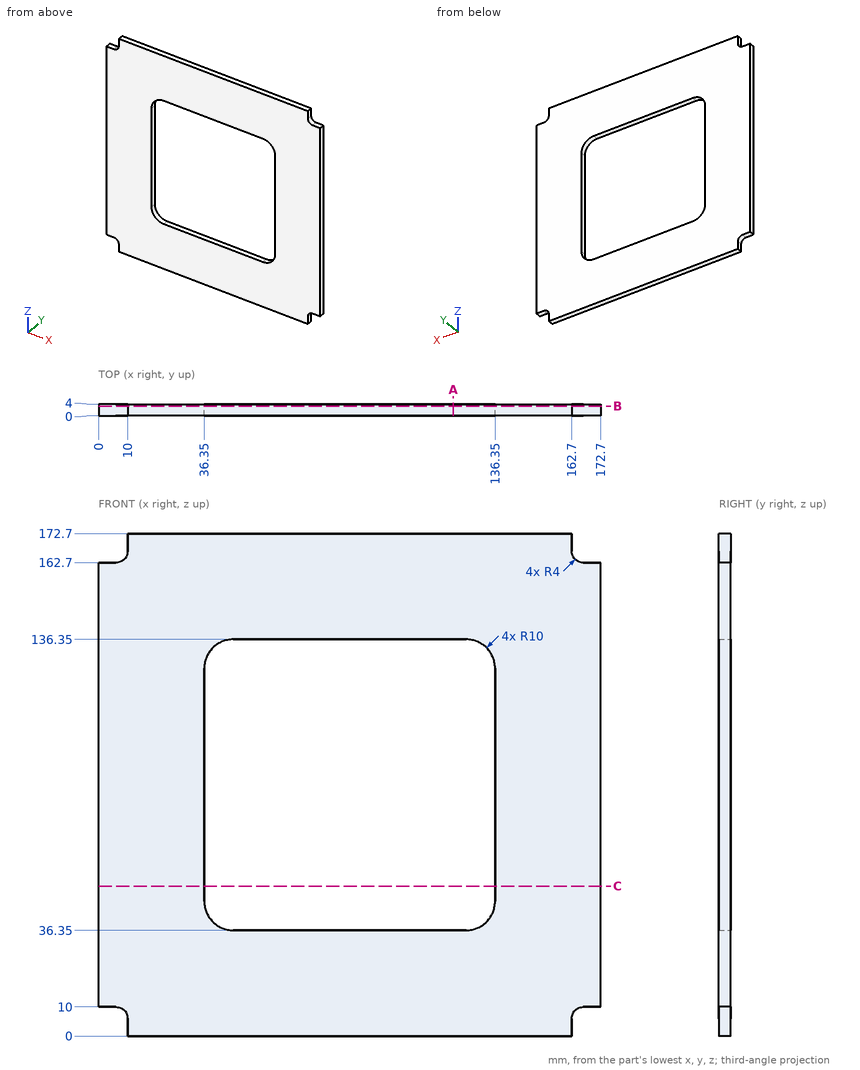
Verification items for this drawing (mm, ordinates from the low corner). Coordinates: 2 decimals unless noted, no trailing zeros. Order: outer loops, then holes, each group sorted by start corner. A loop starts at its lowest first (then second) coordinate and runs counter-clockwise, first axis right, second up. Notation, with made-up numbers: M 44.5,40 L 78.5,40 A25 cw 78.5,78 Z; hole C -4.75,66 d8. An arc over 180 degrees is marked long. One line per item, written item: value. Start each with the question number.
Item 1: Thickness scan on probe 1 along X at (y, z) = (3.35, 97); probe 2 along Z at (x, y) = (42, 2.2). Record the ranges inside material, lowest first.
Item 2: Sectioned sample at C-C on z = 51.5. Record the cut outline in (x, y), then the cut area to 3 significant figures.
Item 3: Sectioned sample at A-A on x = 122. Record the cut outline in (y, z), then the cut area to 3 significant figures.
Item 4: Sectioned sample at B-B on y = 3.3. Record the cut outline in (x, z).
Item 5: Depth check by flat-ended pin: P1, Ø1.2, axis at x = 2.5, y = 1, coming from the +Z side. Enter the tip coordinate at first touch or a pass-through.
Calculated:
1. probe 1: 0 to 36.35, 136.35 to 172.7
1. probe 2: 0 to 37.35, 135.35 to 172.7
2. outline: M 0,0 L 36.35,0 L 36.35,4 L 0,4 Z; M 136.35,0 L 172.7,0 L 172.7,4 L 136.35,4 Z
2. area: 291 mm^2
3. outline: M 0,0 L 4,0 L 4,36.35 L 0,36.35 Z; M 0,136.35 L 4,136.35 L 4,172.7 L 0,172.7 Z
3. area: 291 mm^2
4. outline: M 0,10 L 6,10 A4 cw 10,6 L 10,0 L 162.7,0 L 162.7,6 A4 cw 166.7,10 L 172.7,10 L 172.7,162.7 L 166.7,162.7 A4 cw 162.7,166.7 L 162.7,172.7 L 10,172.7 L 10,166.7 A4 cw 6,162.7 L 0,162.7 Z; hole M 36.35,46.35 A10 ccw 46.35,36.35 L 126.35,36.35 A10 ccw 136.35,46.35 L 136.35,126.35 A10 ccw 126.35,136.35 L 46.35,136.35 A10 ccw 36.35,126.35 Z
5. P1: z = 162.7
